from build123d import *

# Parameters (mm, degrees)
SKETCH1_W           = 30
SKETCH1_H           = 30.000023288
BOSS_EXTRUDE2_DEPTH = 32
FILLET1_R           = 3
SKETCH3_R           = 2.15
CUT_EXTRUDE1_DEPTH  = 63
SKETCH5_W           = 78.057106385
SKETCH5_H           = 38.470116024
CUT_EXTRUDE2_DEPTH  = 63


with BuildPart() as part:
    # Sketch1 → Boss-Extrude2 (new body)
    with BuildSketch(Plane(origin=(0, 0, 0), x_dir=(1, 0, 0), z_dir=(0, 1, 0))):
        Polygon((-15, 15.000011644), (-15, -15.000011644), (-30, -0.01868994), align=None)
        Rectangle(SKETCH1_W, SKETCH1_H)
        Polygon((30, -0.01868994), (15, -15.000011644), (15, 15.000011644), align=None)
    extrude(amount=BOSS_EXTRUDE2_DEPTH)

    # Fillet1
    fillet1_edges = [part.edges().sort_by_distance(p)[0] for p in [
        (-22.5, 0, 7.509350792),
        (-30, 16, 0.01868994),
        (30, 16, 0.01868994),
        (22.5, 32, 7.509350792),
        (22.5, 32, -7.490660852),
        (-22.5, 32, -7.490660852),
        (-22.5, 32, 7.509350792),
        (-22.5, 0, -7.490660852),
        (22.5, 0, -7.490660852),
        (22.5, 0, 7.509350792),
    ]]
    fillet(fillet1_edges, radius=FILLET1_R)

    # Sketch3 → Cut-Extrude1 (cut)
    with BuildSketch(Plane(origin=(0, 32, 0), x_dir=(1, 0, 0), z_dir=(0, 1, 0))):
        with Locations(Location((-7.499998545, -0.004672484, 0), (0, 0, 270))):
            Circle(SKETCH3_R)
        with Locations(Location((7.5, 0.004672485, 0), (0, 0, 270))):
            Circle(SKETCH3_R)
    extrude(amount=-CUT_EXTRUDE1_DEPTH, mode=Mode.SUBTRACT)

    # Sketch5 → Cut-Extrude2 (cut)
    with BuildSketch(Plane.XY):
        with Locations((3.040380137, 18.388870108)):
            Rectangle(SKETCH5_W, SKETCH5_H)
    extrude(amount=-CUT_EXTRUDE2_DEPTH, mode=Mode.SUBTRACT)


solid = part.part
Verification items for the finished model (mm, model axes). Coordinates: 2 decimals unless noted, no trailing zeros. Loops run counter-clockwise (first coordinate to the right, second up) from the corner with the lowest first, then second, coordinate; pieces in that order, holes last. Notation, with made-up numbers: M 23.25,4.5 L 75.25,4.5 A13 ccw 75.25,22.5 Z; hole C 89,-16.5 d8. An arc over 180 degrees is marked long. One line per item, written item: value.
1. Mould release check, pull along X, two halves, no side actions. Record for faces 1 (the flat face through (0, 16, 0)), 2 (the cylindrical face through (-7.547, 16.224, 2.154)), 3 (the cylindrical face through (28.54, 16.18, 1.14)): pulls with the +X half, pulls with the -X half, needs draft (parallel to the pull), parting line crosses it, or undercut.
Answers follow:
face 1: needs draft
face 2: undercut
face 3: pulls with the +X half
2. Gauge pin test, flat ends, axial feed: P1, Ø3, axis at y = 13, z = 12, coming from the -X side; P2, Ø5, axis at y = 21, z = 6, coming from the -X side; P3, Ø1, axis at y = 15.5, z = 1.5, coming from the -X side. Record the tip position at first contact, or that the pin passes through.
Answers follow:
P1: x = -19.51
P2: x = -26.51
P3: x = -28.59
3. Section check B-B on x = -7.5. Record the cut outline in (y, z).
Answers follow:
outline: M 0,2.15 L 32,2.15 L 32,15 L 0,15 Z
4. Section check C-C on z = 1. Give the number of separate pieces and of enclosed holes in the cut face, plus the area to 3 significant figures.
Answers follow:
separate pieces: 3
enclosed holes: 0
area: 1,580 mm^2
5. Material ranges on line 1 along X through (y, z) = (26.5, 1.5); line 2 along Y through (x, z) = (-18, 8); line 3 along X through (y, z) = (8, 5.75), recorded low to high. Write a range as from..to.
Answers follow:
line 1: -28.36..-9.04, -5.96..5.96, 9.04..28.36
line 2: 0..32
line 3: -24.26..24.26
6. Section check A-A on y = 6. Record the cut outline in (x, z).
Answers follow:
outline: M -28.76,0 L -9.65,0 A2.15 cw -5.35,0 L 5.35,0 A2.15 cw 9.65,0 L 28.76,0 A3 ccw 27.88,2.14 L 15,15 L -15,15 L -27.88,2.14 A3 ccw Z
